Verification items for the finished model (mm, model axes). Face numbers are marked on the shaded views. A direction names the side the tool comes from. Give positions to 0.01 mm unless a question says otherwise; leave off trailing zeros. Order: outer loops, then holes, each group sorted by start corner. A loop starts at its lowest first (then second) coordinate and runs counter-clockwise, first axis right, second up. Notation, with made-up numbers: (26.5, 81) -> (56.5, 81) arc R15 cw to (56.5, 109) -> close; hole circle Ø5 at (-21, 2.25). An arc over 180 degrees is marked (long way). One line per question, with ' | ' between items. Start each with the question number.
Q1. Go/stop test with flat-tipped pins: pin 1 (1.8 mm diameter, centred on y = 13.5, z = -0.5, fed in from +X); pin 2 (1 mm diameter, centred on x = -6, y = -9.5, fed in from -Z); pin 3 (1 mm diameter, centred on x = 16, z = 1, fed in from +Y). Record where each tip stops, or that it passes through.
Q2. Mould release check, pull along X, two halves, no side actions. Record for the marked faces 5, 6 and 7: released by +X, released by -X, zero draft, split by the parting line, or undercut.
Q3. Section check B-B on y = -13.5. Record the cut outline in (x, z), plus the area to 3 significant figures.
Q4. Section check D-D on y = -6.5. Record the cut outline in (x, z).
Q5. Access from +Z, -Z, +X, -X, +Y, -Y to the whole of each face (thin tool, end or side, straight path). Record for the marked faces 1, 2, 3 and 4.
Q6. Section check A-A on x = -5.5. Record the cut outline in (y, z).
Q7. Section check C-C on z = -0.3. Record the cut outline in (x, y), plus the area to 3 significant figures.
Q8. Material ranges on probe 1 along X at (y, z) = (15, -1.1); probe 2 along Y at (x, z) = (-1, -1.3); probe 3 along Y at (x, z) = (-5, 1.75), recorded low to high. Write a range as [from, to].
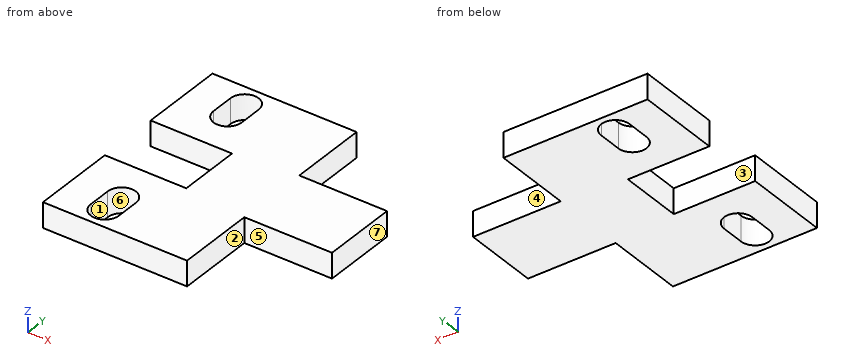
from build123d import *

# Parameters (mm, degrees)
BOSS_EXTRUDE1_DEPTH      = 2
M4_START                 = -2
M4_CLEARANCE_SLOT1_DEPTH = 4


# Read off the part's stored shape, not the designer's step: M4 Clearance Slot1
with BuildPart() as part:
    # Sketch1 → Boss-Extrude1 (new, symmetric)
    with BuildSketch(Plane.XY):
        Polygon((0, 0), (0, -5), (-13, -5), (-13, -18.5), (10, -18.5), (10, -6), (24, -6), (24, 0), align=None)
    boss_extrude1 = extrude(amount=BOSS_EXTRUDE1_DEPTH, both=True)

    # M4 Clearance Slot1 outline → M4 Clearance Slot1 (cut)
    with BuildSketch(Plane.XY.offset(M4_START)):
        with BuildLine():
            Line((-7.75, -11.55), (-7.75, -15.25))
            ThreePointArc((-7.75, -15.25), (-5.5, -17.5), (-3.25, -15.25))
            Line((-3.25, -15.25), (-3.25, -11.55))
            ThreePointArc((-3.25, -11.55), (-5.5, -9.3), (-7.75, -11.55))
        make_face()
    m4_clearance_slot1 = extrude(amount=M4_CLEARANCE_SLOT1_DEPTH, mode=Mode.SUBTRACT)

    # Mirror2: Boss-Extrude1, M4 Clearance Slot1 across plane
    add(boss_extrude1.mirror(Plane.ZX))
    add(m4_clearance_slot1.mirror(Plane.ZX), mode=Mode.SUBTRACT)


solid = part.part
Filled in:
1) pin 1: x = 10 | pin 2: z = -2 | pin 3: y = 6
2) face 5: zero draft | face 6: undercut | face 7: released by +X
3) outline: (-13, -2) -> (-7.75, -2) -> (-7.75, 2) -> (-13, 2) -> close; (-3.25, -2) -> (10, -2) -> (10, 2) -> (-3.25, 2) -> close | area: 74.0 mm²
4) outline: (-13, -2) -> (10, -2) -> (10, 2) -> (-13, 2) -> close
5) face 1: +Z, -Z | face 2: +Z, -Z, +X, -Y | face 3: +Z, -Z, -X | face 4: +Z, -Z, +X, +Y
6) outline: (-18.5, -2) -> (-17.5, -2) -> (-17.5, 2) -> (-18.5, 2) -> close; (-9.3, -2) -> (-5, -2) -> (-5, 2) -> (-9.3, 2) -> close; (5, -2) -> (9.3, -2) -> (9.3, 2) -> (5, 2) -> close; (17.5, -2) -> (18.5, -2) -> (18.5, 2) -> (17.5, 2) -> close
7) outline: (-13, -18.5) -> (10, -18.5) -> (10, -6) -> (24, -6) -> (24, 6) -> (10, 6) -> (10, 18.5) -> (-13, 18.5) -> (-13, 5) -> (0, 5) -> (0, -5) -> (-13, -5) -> close; hole (-7.75, -15.25) arc R2.25 ccw to (-3.25, -15.25) -> (-3.25, -11.55) arc R2.25 ccw to (-7.75, -11.55) -> close; hole (-7.75, 11.55) arc R2.25 ccw to (-3.25, 11.55) -> (-3.25, 15.25) arc R2.25 ccw to (-7.75, 15.25) -> close | area: 824 mm²
8) probe 1: [-13, -7.75], [-3.25, 10] | probe 2: [-18.5, -5], [5, 18.5] | probe 3: [-18.5, -17.44], [-9.36, -5], [5, 9.36], [17.44, 18.5]
